from build123d import *

# Parameters (mm, degrees)
SKETCH4_R                = 5
BOSS_EXTRUDE2_DEPTH      = 17.5
BOSS_EXTRUDE2_DEPTH_BACK = 17.5
SKETCH7_W                = 20
SKETCH7_H                = 2.5
SKETCH8_R                = 5
CUT_EXTRUDE1_DEPTH       = 18.5
CUT_EXTRUDE1_DEPTH_BACK  = 18.6


with BuildPart() as part:
    # Sweep-Thin1: sweep along a path in Sketch1
    with BuildLine(Plane(origin=(0, 0, 0), x_dir=(1, 0, 0), z_dir=(0, 1, 0))) as sweep_thin1_path:
        Line((0, 0), (330, 0))
        ThreePointArc((330, 0), (344.142135624, -5.857864376), (350, -20))
        Line((350, -20), (350, -395))
    # Sketch2 → Sweep-Thin1 (sweep)
    with BuildSketch(Plane(origin=(0, 0, 0), x_dir=(0, 0, -1), z_dir=(1, 0, 0))):
        with BuildLine():
            Line((1.5, 9.5), (-1.5, 9.5))
            ThreePointArc((-1.5, 9.5), (-7.156854249, 7.156854249), (-9.5, 1.5))
            Line((-9.5, 1.5), (-9.5, -1.5))
            ThreePointArc((-9.5, -1.5), (-7.156854249, -7.156854249), (-1.5, -9.5))
            Line((-1.5, -9.5), (1.5, -9.5))
            ThreePointArc((1.5, -9.5), (7.156854249, -7.156854249), (9.5, -1.5))
            Line((9.5, -1.5), (9.5, 1.5))
            ThreePointArc((9.5, 1.5), (7.156854249, 7.156854249), (1.5, 9.5))
        make_face()
        with BuildLine():
            Line((1.5, 6.5), (-1.5, 6.5))
            ThreePointArc((-1.5, 6.5), (-5.035533906, 5.035533906), (-6.5, 1.5))
            Line((-6.5, 1.5), (-6.5, -1.5))
            ThreePointArc((-6.5, -1.5), (-5.035533906, -5.035533906), (-1.5, -6.5))
            Line((-1.5, -6.5), (1.5, -6.5))
            ThreePointArc((1.5, -6.5), (5.035533906, -5.035533906), (6.5, -1.5))
            Line((6.5, -1.5), (6.5, 1.5))
            ThreePointArc((6.5, 1.5), (5.035533906, 5.035533906), (1.5, 6.5))
        make_face(mode=Mode.SUBTRACT)
    sweep(path=sweep_thin1_path.line)



with BuildPart() as body_2:
    # Sketch4 → Boss-Extrude2 (new body, two sides)
    with BuildSketch(Plane(origin=(0, 0, 0), x_dir=(1, 0, 0), z_dir=(0, 1, 0))) as boss_extrude2_sk:
        with Locations((350, -450)):
            Circle(SKETCH4_R)
    extrude(amount=BOSS_EXTRUDE2_DEPTH)
    extrude(boss_extrude2_sk.sketch, amount=-BOSS_EXTRUDE2_DEPTH_BACK)


with BuildPart() as part_1:
    add(part.part)

    add(body_2.part)  # Sweep1 merges body 2
    # Sweep1: sweep along a path in Sketch6
    with BuildLine(Plane(origin=(350, 0, 0), x_dir=(0, 0, -1), z_dir=(1, 0, 0))) as sweep1_path:
        Line((-460, 17.4), (-395, 17.4))
        Line((-395, 17.4), (-395, 0))
        Line((-395, 0), (-395, -15.485164569))
        Line((-395, -15.485164569), (-460, -17.6))
    # Sketch7 → Sweep1 (sweep)
    with BuildSketch(Plane.XY.offset(460)):
        with Locations((350, -16.35)):
            Rectangle(SKETCH7_W, SKETCH7_H)
    sweep(path=sweep1_path.line, transition=Transition.RIGHT)

    # Sketch8 → Cut-Extrude1 (cut, two sides)
    with BuildSketch(Plane(origin=(0, 0, 0), x_dir=(1, 0, 0), z_dir=(0, 1, 0))) as cut_extrude1_sk:
        with Locations((30, 0)):
            Circle(SKETCH8_R)
    extrude(amount=CUT_EXTRUDE1_DEPTH, mode=Mode.SUBTRACT)
    extrude(cut_extrude1_sk.sketch, amount=-CUT_EXTRUDE1_DEPTH_BACK, mode=Mode.SUBTRACT)


solid = part_1.part
Work out the finished part from the listing and answer in its coordinate system (mm). A direction names the side the tool comes from. Give positions to 0.01 mm unless a question says otherwise; leave off trailing zeros. Write each loop counter-clockwise with the first axis right and the second up, starting at its lowest first coordinate (ties: lowest second). Pieces come first, ordered by that corner, then holes.
Q1. Given pin 1 (6 mm diameter, centred on x = 350.5, y = 5.5, fed in from +Z); pin 2 (10 mm diameter, centred on x = 220.5, y = 0.5, fed in from +Z); pin 3 (11.5 mm diameter, centred on x = 30, z = 0, fed in from -Y), each flat-ended and moving along its own axis, determine where each tip first touches the part or whether it passes through.
Answer:
pin 1: stops at z = 455
pin 2: stops at z = 9.5
pin 3: stops at y = -9.5
Q2. For a pull along Y with two mould halves and no side action, classify faces 5 (the face through (353, 0, 446)), 6 (the face through (350, -17.5, 450)), 7 (the face through (360, -14, 418)), 8 (the face through (350, 17.5, 450)) as released by +Y, released by -Y, zero draft, split by the parting line, or undercut.
Answer:
face 5: undercut
face 6: released by -Y
face 7: zero draft
face 8: released by +Y
Q3. Straight lines are drawn through the part: L1, parallel to Z at x = 195, y = 1; L2, parallel to Z at x = 299, y = -2.5; L3, parallel to Y at x = 345.5, z = 263. For each, find the intervals that lie inside material, in ascending order.
Answer:
L1: z = -9.5 to -6.5, 6.5 to 9.5
L2: z = -9.44 to -6.4, 6.4 to 9.44
L3: y = -8.92 to -5.5, 5.5 to 8.92
Q4. The part is cut by section B-B on z = 213.5. Give the vertices of the cut face in (x, y), and give its area (3 significant figures).
Answer:
outline: (340.5, -1.5) arc R8 ccw to (348.5, -9.5) - (351.5, -9.5) arc R8 ccw to (359.5, -1.5) - (359.5, 1.5) arc R8 ccw to (351.5, 9.5) - (348.5, 9.5) arc R8 ccw to (340.5, 1.5) - close; hole (343.5, -1.5) arc R5 ccw to (348.5, -6.5) - (351.5, -6.5) arc R5 ccw to (356.5, -1.5) - (356.5, 1.5) arc R5 ccw to (351.5, 6.5) - (348.5, 6.5) arc R5 ccw to (343.5, 1.5) - close
area: 159 mm2
Q5. A tool of negligible diameter and unlimited length cuts with its end or side. For faces 1 (the face through (350.629, 0.021, -1.088)), 2 (the face through (337.34, -0.02, 12.49)), 3 (the face through (350, 1, 397.499)), 4 (the face through (350, 0, 395)), from which of +Z, -Z, +X, -X, +Y, -Y can it reach the whole face along a straight path? Write none if from no direction.
Answer:
face 1: -Z, +X, +Y, -Y
face 2: -X, +Y, -Y
face 3: +X, -X
face 4: none
Q6. The part is cut by section C-C on x = 30. Give the vertices of the cut face in (y, z).
Answer:
outline: (-8.69, -5) arc R8 ccw to (-1.5, -9.5) - (1.5, -9.5) arc R8 ccw to (8.69, -5) - (5.07, -5) arc R5 cw to (1.5, -6.5) - (-1.5, -6.5) arc R5 cw to (-5.07, -5) - close; (-8.69, 5) - (-5.07, 5) arc R5 cw to (-1.5, 6.5) - (1.5, 6.5) arc R5 cw to (5.07, 5) - (8.69, 5) arc R8 ccw to (1.5, 9.5) - (-1.5, 9.5) arc R8 ccw to start
Q7. The part is cut by section A-A on x = 118. Give the vertices of the cut face in (y, z).
Answer:
outline: (-9.5, -1.5) arc R8 ccw to (-1.5, -9.5) - (1.5, -9.5) arc R8 ccw to (9.5, -1.5) - (9.5, 1.5) arc R8 ccw to (1.5, 9.5) - (-1.5, 9.5) arc R8 ccw to (-9.5, 1.5) - close; hole (-6.5, -1.5) arc R5 ccw to (-1.5, -6.5) - (1.5, -6.5) arc R5 ccw to (6.5, -1.5) - (6.5, 1.5) arc R5 ccw to (1.5, 6.5) - (-1.5, 6.5) arc R5 ccw to (-6.5, 1.5) - close
